from build123d import *

# Parameters (mm, degrees)
SKETCH1_W           = 12.5
SKETCH1_H           = 22.5
BOSS_EXTRUDE1_DEPTH = 19
SKETCH2_W           = 12.5
SKETCH2_H           = 32.1
BOSS_EXTRUDE2_DEPTH = 2.5
SKETCH3_W           = 12.5
SKETCH3_H           = 22.5
BOSS_EXTRUDE3_DEPTH = 3.9
BOSS_EXTRUDE4_DEPTH = 4.2
BOSS_EXTRUDE5_DEPTH = 3
CUT_EXTRUDE1_DEPTH  = 20


with BuildPart() as part:
    # Sketch1 → Boss-Extrude1 (new body)
    with BuildSketch(Plane(origin=(0, 0, 0), x_dir=(1, 0, 0), z_dir=(0, 1, 0))):
        Rectangle(SKETCH1_W, SKETCH1_H)
    extrude(amount=BOSS_EXTRUDE1_DEPTH)

    # Sketch2 → Boss-Extrude2 (add)
    with BuildSketch(Plane(origin=(0, 19, 0), x_dir=(1, 0, 0), z_dir=(0, 1, 0))):
        Rectangle(SKETCH2_W, SKETCH2_H)
    extrude(amount=-BOSS_EXTRUDE2_DEPTH)

    # Sketch3 → Boss-Extrude3 (add)
    with BuildSketch(Plane(origin=(0, 19, 0), x_dir=(1, 0, 0), z_dir=(0, 1, 0))):
        Rectangle(SKETCH3_W, SKETCH3_H)
    extrude(amount=BOSS_EXTRUDE3_DEPTH)

    # Sketch4 → Boss-Extrude4 (add)
    with BuildSketch(Plane(origin=(0, 22.9, 0), x_dir=(1, 0, 0), z_dir=(0, 1, 0))):
        with BuildLine():
            ThreePointArc((-2.75, 0.61248608), (0, -11.25), (2.75, 0.61248608))
            ThreePointArc((2.75, 0.61248608), (0, 3.25), (-2.75, 0.61248608))
        make_face()
    extrude(amount=BOSS_EXTRUDE4_DEPTH)

    # Sketch5 → Boss-Extrude5 (add)
    with BuildSketch(Plane(origin=(0, 27.1, 0), x_dir=(1, 0, 0), z_dir=(0, 1, 0))):
        with BuildLine():
            ThreePointArc((-0.25, -2.613056348), (-0.250868312, -2.613147451), (-0.25173659, -2.613238871))
            ThreePointArc((-0.25173659, -2.613238871), (-0.485877906, -2.714124173), (-0.740810391, -2.717194716))
            ThreePointArc((-0.740810391, -2.717194716), (-0.741640786, -2.717464361), (-0.742471084, -2.717734308))
            ThreePointArc((-0.742471084, -2.717734308), (-0.950520616, -2.865095742), (-1.199243813, -2.921102629))
            ThreePointArc((-1.199243813, -2.921102629), (-1.2, -2.921539031), (-1.200756028, -2.921975707))
            ThreePointArc((-1.200756028, -2.921975707), (-1.373621014, -3.10937287), (-1.605264526, -3.215868334))
            ThreePointArc((-1.605264526, -3.215868334), (-1.605913455, -3.216452419), (-1.606562172, -3.21703674))
            ThreePointArc((-1.606562172, -3.21703674), (-1.736687583, -3.436279477), (-1.941127476, -3.588609153))
            ThreePointArc((-1.941127476, -3.588609153), (-1.941640786, -3.589315394), (-1.94215384, -3.590021823))
            ThreePointArc((-1.94215384, -3.590021823), (-2.02385257, -3.831528174), (-2.19215384, -4.023034525))
            ThreePointArc((-2.19215384, -4.023034525), (-2.192509098, -4.023832057), (-2.192864066, -4.024629718))
            ThreePointArc((-2.192864066, -4.024629718), (-2.222565489, -4.277844696), (-2.347372563, -4.500157976))
            ThreePointArc((-2.347372563, -4.500157976), (-2.347554242, -4.501011942), (-2.34773561, -4.501865974))
            ThreePointArc((-2.34773561, -4.501865974), (-2.324141631, -4.755722871), (-2.399999841, -4.999126922))
            ThreePointArc((-2.399999841, -4.999126922), (-2.4, -5), (-2.399999841, -5.000873078))
            ThreePointArc((-2.399999841, -5.000873078), (-2.324141631, -5.244277129), (-2.34773561, -5.498134026))
            ThreePointArc((-2.34773561, -5.498134026), (-2.347554242, -5.498988058), (-2.347372563, -5.499842024))
            ThreePointArc((-2.347372563, -5.499842024), (-2.222565489, -5.722155304), (-2.192864066, -5.975370282))
            ThreePointArc((-2.192864066, -5.975370282), (-2.192509098, -5.976167943), (-2.19215384, -5.976965475))
            ThreePointArc((-2.19215384, -5.976965475), (-2.02385257, -6.168471826), (-1.94215384, -6.409978177))
            ThreePointArc((-1.94215384, -6.409978177), (-1.941640786, -6.410684606), (-1.941127476, -6.411390847))
            ThreePointArc((-1.941127476, -6.411390847), (-1.736687583, -6.563720523), (-1.606562172, -6.78296326))
            ThreePointArc((-1.606562172, -6.78296326), (-1.605913455, -6.783547581), (-1.605264526, -6.784131666))
            ThreePointArc((-1.605264526, -6.784131666), (-1.373621014, -6.89062713), (-1.200756028, -7.078024293))
            ThreePointArc((-1.200756028, -7.078024293), (-1.2, -7.078460969), (-1.199243813, -7.078897371))
            ThreePointArc((-1.199243813, -7.078897371), (-0.950520616, -7.134904258), (-0.742471084, -7.282265692))
            ThreePointArc((-0.742471084, -7.282265692), (-0.741640786, -7.282535639), (-0.740810391, -7.282805284))
            ThreePointArc((-0.740810391, -7.282805284), (-0.485877906, -7.285875827), (-0.25173659, -7.386761129))
            ThreePointArc((-0.25173659, -7.386761129), (-0.250868312, -7.386852549), (-0.25, -7.386943652))
            ThreePointArc((-0.25, -7.386943652), (0, -7.336943652), (0.25, -7.386943652))
            ThreePointArc((0.25, -7.386943652), (0.250868312, -7.386852549), (0.25173659, -7.386761129))
            ThreePointArc((0.25173659, -7.386761129), (0.485877906, -7.285875827), (0.740810391, -7.282805284))
            ThreePointArc((0.740810391, -7.282805284), (0.741640786, -7.282535639), (0.742471084, -7.282265692))
            ThreePointArc((0.742471084, -7.282265692), (0.950520616, -7.134904258), (1.199243813, -7.078897371))
            ThreePointArc((1.199243813, -7.078897371), (1.2, -7.078460969), (1.200756028, -7.078024293))
            ThreePointArc((1.200756028, -7.078024293), (1.373621014, -6.89062713), (1.605264526, -6.784131666))
            ThreePointArc((1.605264526, -6.784131666), (1.605913455, -6.783547581), (1.606562172, -6.78296326))
            ThreePointArc((1.606562172, -6.78296326), (1.736687583, -6.563720523), (1.941127476, -6.411390847))
            ThreePointArc((1.941127476, -6.411390847), (1.941640786, -6.410684606), (1.94215384, -6.409978177))
            ThreePointArc((1.94215384, -6.409978177), (2.02385257, -6.168471826), (2.19215384, -5.976965475))
            ThreePointArc((2.19215384, -5.976965475), (2.192509098, -5.976167943), (2.192864066, -5.975370282))
            ThreePointArc((2.192864066, -5.975370282), (2.222565489, -5.722155304), (2.347372563, -5.499842024))
            ThreePointArc((2.347372563, -5.499842024), (2.347554242, -5.498988058), (2.34773561, -5.498134026))
            ThreePointArc((2.34773561, -5.498134026), (2.324141631, -5.244277129), (2.399999841, -5.000873078))
            ThreePointArc((2.399999841, -5.000873078), (2.4, -5), (2.399999841, -4.999126922))
            ThreePointArc((2.399999841, -4.999126922), (2.324141631, -4.755722871), (2.34773561, -4.501865974))
            ThreePointArc((2.34773561, -4.501865974), (2.347554242, -4.501011942), (2.347372563, -4.500157976))
            ThreePointArc((2.347372563, -4.500157976), (2.222565489, -4.277844696), (2.192864066, -4.024629718))
            ThreePointArc((2.192864066, -4.024629718), (2.192509098, -4.023832057), (2.19215384, -4.023034525))
            ThreePointArc((2.19215384, -4.023034525), (2.02385257, -3.831528174), (1.94215384, -3.590021823))
            ThreePointArc((1.94215384, -3.590021823), (1.941640786, -3.589315394), (1.941127476, -3.588609153))
            ThreePointArc((1.941127476, -3.588609153), (1.736687583, -3.436279477), (1.606562172, -3.21703674))
            ThreePointArc((1.606562172, -3.21703674), (1.605913455, -3.216452419), (1.605264526, -3.215868334))
            ThreePointArc((1.605264526, -3.215868334), (1.373621014, -3.10937287), (1.200756028, -2.921975707))
            ThreePointArc((1.200756028, -2.921975707), (1.2, -2.921539031), (1.199243813, -2.921102629))
            ThreePointArc((1.199243813, -2.921102629), (0.950520616, -2.865095742), (0.742471084, -2.717734308))
            ThreePointArc((0.742471084, -2.717734308), (0.741640786, -2.717464361), (0.740810391, -2.717194716))
            ThreePointArc((0.740810391, -2.717194716), (0.485877906, -2.714124173), (0.25173659, -2.613238871))
            ThreePointArc((0.25173659, -2.613238871), (0.250868312, -2.613147451), (0.25, -2.613056348))
            ThreePointArc((0.25, -2.613056348), (0, -2.663056348), (-0.25, -2.613056348))
        make_face()
    extrude(amount=BOSS_EXTRUDE5_DEPTH)

    # Sketch6 → Cut-Extrude1 (cut, through all)
    with BuildSketch(Plane(origin=(0, 19, 0), x_dir=(1, 0, 0), z_dir=(0, 1, 0))):
        with BuildLine():
            Line((0.5, 16.05), (0.5, 15.05))
            ThreePointArc((0.5, 15.05), (0, 12.135786438), (-0.5, 15.05))
            Line((-0.5, 15.05), (-0.5, 16.05))
            Line((-0.5, 16.05), (0.5, 16.05))
        make_face()
        with BuildLine():
            Line((-0.5, -16.05), (-0.5, -15.05))
            ThreePointArc((-0.5, -15.05), (0, -12.135786438), (0.5, -15.05))
            Line((0.5, -15.05), (0.5, -16.05))
            Line((0.5, -16.05), (-0.5, -16.05))
        make_face()
    extrude(amount=-CUT_EXTRUDE1_DEPTH, mode=Mode.SUBTRACT)


solid = part.part
For this review, take the finished solid that the model builds, in its own axes (mm). A direction names the side the tool comes from. Give positions to 0.01 mm unless a question says otherwise; leave off trailing zeros. Loops run counter-clockwise (first coordinate to the right, second up) from the corner with the lowest first, then second, coordinate; pieces in that order, holes last.
Item 1: Tool access review of faces 5 (the flat face through (0, 8, -11.25)), 6 (the flat face through (5, 22.9, 10)), 7 (the flat face through (-0.5, 17.8, -15.5)), 8 (the flat face through (-1.5, 19, -12.6)), 9 (the flat face through (-5, 22.9, 10)): name each direction out of +Z, -Z, +X, -X, +Y, -Y from which nothing blocks a thin tool from reaching the whole face with its end or side.
Item 2: Draft analysis for pull direction X (two halves, no side actions). For faces 1 (the cylindrical face through (0.059, 17.768, -12.137)), 2 (the flat face through (3, 18, -16.05)), 3 (the cylindrical face through (-0.235, 24.971, 11.246)), 4 (the flat face through (0.5, 17.8, 15.5)), state which applies: +X half, -X half, draft (parallel to the pull), parting line (faces both ways), or undercut.
Item 3: Take a section at C-C, the plane x = -4.5. State the section outline as (y, z) points.
Item 4: Take a section at D-D, the plane z = 1.5. State the section outline as (x, y) points.
Item 5: Take a section at A-A, the plane y = 17.5. State the section outline as (x, z) points.
Item 6: For line 1 along Y through (x, z) = (3.5, 2.5); line 2 along Y through (x, z) = (-4.5, -4); line 3 along Z through (x, y) = (-3.5, 19.5), list the stretches that pass through material, from the lowest coordinate up.
Item 7: Insertion check: pin 1 (6 mm diameter, centred on x = 0.5, y = 6.5, fed in from +Z); pin 2 (2.5 mm diameter, centred on x = -3, z = 14.5, fed in from -Y); pin 3 (4 mm diameter, centred on x = -1, z = -15, fed in from +Y); pin 4 (1.8 mm diameter, centred on x = 0, z = 13.64, fed in from -Y). Each pin has a flat end and moves straight along its axis. Give the tip position at first contact, or say it passes through.
Item 8: Take a section at B-B, the plane z = -4. State the section outline as (x, y) points.
Calculated:
1. face 5: -Z, +X, -X, -Y
1. face 6: +Z, +X, +Y
1. face 7: -Z, +Y, -Y
1. face 8: -Z, +X, -X, +Y
1. face 9: +Z, -X, +Y
2. face 1: undercut
2. face 2: draft
2. face 3: parting line
2. face 4: undercut
3. outline: (0, -11.25) - (16.5, -11.25) - (16.5, -16.05) - (19, -16.05) - (19, -11.25) - (22.9, -11.25) - (22.9, 0.66) - (27.1, 0.66) - (27.1, 9.34) - (22.9, 9.34) - (22.9, 11.25) - (19, 11.25) - (19, 16.05) - (16.5, 16.05) - (16.5, 11.25) - (0, 11.25) - close
4. outline: (-6.25, 0) - (6.25, 0) - (6.25, 22.9) - (5.18, 22.9) - (5.18, 27.1) - (-5.18, 27.1) - (-5.18, 22.9) - (-6.25, 22.9) - close
5. outline: (-6.25, -16.05) - (-0.5, -16.05) - (-0.5, -15.05) arc R1.5 cw (long way) to (0.5, -15.05) - (0.5, -16.05) - (6.25, -16.05) - (6.25, 16.05) - (0.5, 16.05) - (0.5, 15.05) arc R1.5 cw (long way) to (-0.5, 15.05) - (-0.5, 16.05) - (-6.25, 16.05) - close
6. line 1: y = 0 to 27.1
6. line 2: y = 0 to 22.9
6. line 3: z = -11.25 to 11.25
7. pin 1: stops at z = 11.25
7. pin 2: stops at y = 16.5
7. pin 3: stops at y = 19
7. pin 4: passes through
8. outline: (-6.25, 0) - (6.25, 0) - (6.25, 22.9) - (-6.25, 22.9) - close
